Job drawing, mm, ordinate dimensions from the low corner. One solid piece. A direction names the side the tool comes from. Give positions to 0.01 mm unless a question says otherwise; leave off trailing zeros. Loops run counter-clockwise (first coordinate to the right, second up) from the corner with the lowest first, then second, coordinate; pieces in that order, holes last. Notation, with made-up numbers: (42, 39.5) - (85, 39.5) arc R18 cw to (85, 50.5) - close; hole circle Ø8 at (29.25, 40). An arc over 180 degrees is marked (long way). Use a Markdown table: item, result.
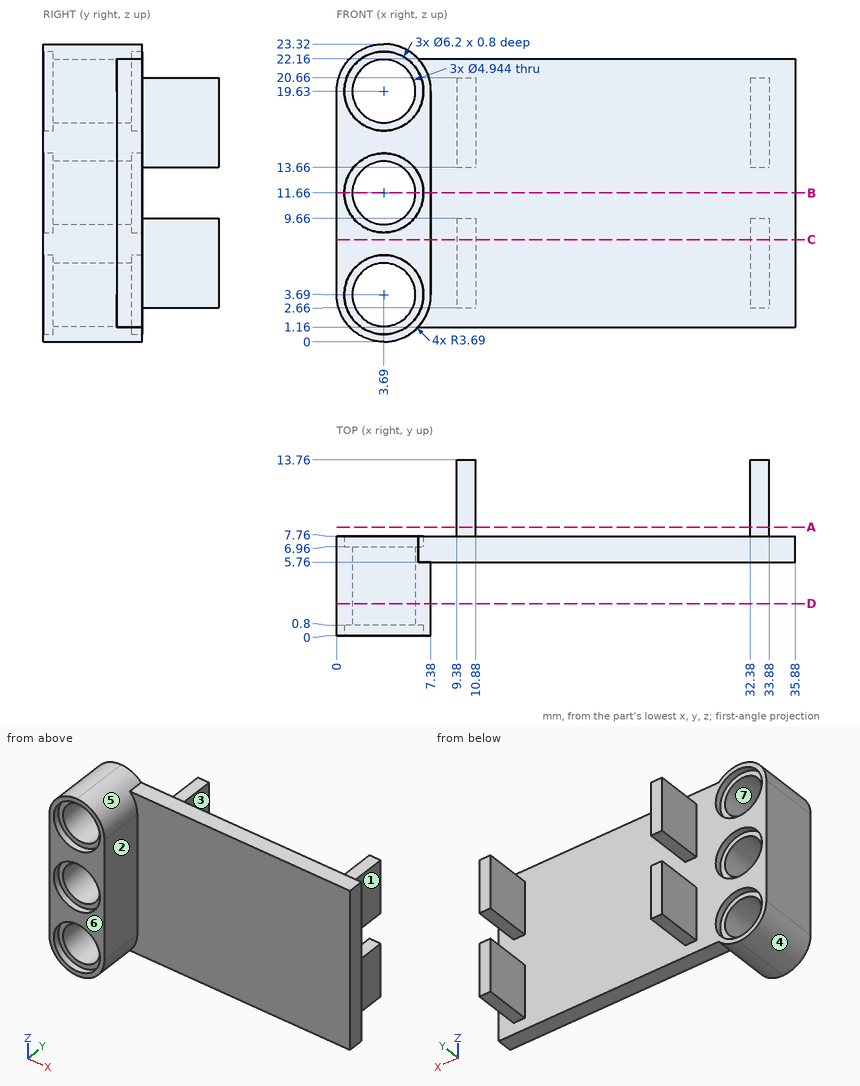
(1) Slice it at C-C, the plane z = 8. Write the cut outline in (x, y), plus the area to 3 significant figures.
Computed:
| item | result |
|---|---|
| outline | (0, 0) - (7.38, 0) - (7.38, 5.76) - (35.88, 5.76) - (35.88, 7.76) - (33.88, 7.76) - (33.88, 13.76) - (32.38, 13.76) - (32.38, 7.76) - (10.88, 7.76) - (10.88, 13.76) - (9.38, 13.76) - (9.38, 7.76) - (0, 7.76) - close |
| area | 132 mm² |
(2) Slice it at B-B, the plane z = 11.66. Write the cut outline in (x, y).
Computed:
| item | result |
|---|---|
| outline | (0, 0) - (0.59, 0) - (0.59, 0.8) - (1.22, 0.8) - (1.22, 6.96) - (0.59, 6.96) - (0.59, 7.76) - (0, 7.76) - close; (6.16, 0.8) - (6.79, 0.8) - (6.79, 0) - (7.38, 0) - (7.38, 5.76) - (35.88, 5.76) - (35.88, 7.76) - (6.79, 7.76) - (6.79, 6.96) - (6.16, 6.96) - close |
(3) Pin check, flat tips, straight feed: P1, Ø1.5, axis at x = 4, z = 7, coming from the +Y side; P2, Ø1.6, axis at x = 33, y = 10, coming from the -Z side; P3, Ø1.8, axis at y = 9.5, z = 16.5, coming from the +X side. Stop position of each tip, or through.
Computed:
| item | result |
|---|---|
| P1 | y = 7.76 |
| P2 | z = 2.66 |
| P3 | x = 33.88 |
(4) Drill centre lines: probe 1 along X at (y, z) = (11.25, 9); probe 2 along Z at (x, y) = (33, 11.5); probe 3 along Z at (x, y) = (2.5, 4.5). Where is each one in solid material? Low to high. Write a range as [from, to].
Computed:
| item | result |
|---|---|
| probe 1 | [9.38, 10.88], [32.38, 33.88] |
| probe 2 | [2.66, 9.66], [13.66, 20.66] |
| probe 3 | [0.2, 1.52], [5.86, 9.49], [13.83, 17.46], [21.8, 23.12] |
(5) Mould opens along Z. For the marked faces 4, 5, 6 and 7 say: pulls with the +Z half, pulls with the -Z half, needs draft (parallel to the pull), parting line crosses it, or undercut.
Computed:
| item | result |
|---|---|
| face 4 | pulls with the -Z half |
| face 5 | pulls with the +Z half |
| face 6 | needs draft |
| face 7 | undercut |
(6) Slice it at D-D, the plane y = 2.5. Count the separate pieces of the cut face and the enclosed holes in it, plus the area to 3 significant figures.
Computed:
| item | result |
|---|---|
| separate pieces | 1 |
| enclosed holes | 3 |
| area | 103 mm² |
(7) Slice it at A-A, the plane y = 8.5. Write the cut outline in (x, z).
Computed:
| item | result |
|---|---|
| outline | (9.38, 2.66) - (10.88, 2.66) - (10.88, 9.66) - (9.38, 9.66) - close; (9.38, 13.66) - (10.88, 13.66) - (10.88, 20.66) - (9.38, 20.66) - close; (32.38, 2.66) - (33.88, 2.66) - (33.88, 9.66) - (32.38, 9.66) - close; (32.38, 13.66) - (33.88, 13.66) - (33.88, 20.66) - (32.38, 20.66) - close |
(8) 3-axis set-ups, long thin cutter, end or side, ignore diameter. For the marked faces 1, 2 and 3: which of +Z, -Z, +X, -X, +Y, -Y reach the whole face in a straight line?
Computed:
| item | result |
|---|---|
| face 1 | +Z, -Z, +X, +Y |
| face 2 | +Z, -Z, +X, -Y |
| face 3 | +Z, -Z, +Y |
